```python
from build123d import *

# Parameters (mm, degrees)
BOSS_EXTRUDE1_DEPTH = 5
SKETCH2_R           = 2
CUT_EXTRUDE1_DEPTH  = 5
FILLET1_R           = 10
FILLET2_R           = 10


with BuildPart() as part:
    # Sketch1 → Boss-Extrude1 (new body)
    with BuildSketch(Plane(origin=(0, 0, 0), x_dir=(0, 0, -1), z_dir=(1, 0, 0))):
        with BuildLine():
            Line((3.89561725, -3.134352603), (36.078990527, 36.865647397))
            ThreePointArc((36.078990527, 36.865647397), (35.317725879, 43.89561725), (28.287756026, 43.134352603))
            Line((28.287756026, 43.134352603), (-3.055770002, 4.178180099))
            Line((-3.055770002, 4.178180099), (-21.704720416, -3.047928704))
            ThreePointArc((-21.704720416, -3.047928704), (-24.560430819, -9.516693509), (-18.091666014, -12.372403912))
            Line((-18.091666014, -12.372403912), (1.806527201, -4.662237604))
            Line((1.806527201, -4.662237604), (3.055770002, -4.178180099))
            Line((3.055770002, -4.178180099), (3.89561725, -3.134352603))
        make_face()
    extrude(amount=BOSS_EXTRUDE1_DEPTH)

    # Sketch2 → Cut-Extrude1 (cut)
    with BuildSketch(Plane(origin=(5, 0, 0), x_dir=(0, 0, -1), z_dir=(1, 0, 0))):
        with Locations((28.965035949, 36)):
            Circle(SKETCH2_R)
        with Locations((19.561978141, 24.313148249)):
            Circle(SKETCH2_R)
        with Locations((10.158920332, 12.626296498)):
            Circle(SKETCH2_R)
        with Locations((0.755862524, 0.939444747)):
            Circle(SKETCH2_R)
    extrude(amount=-CUT_EXTRUDE1_DEPTH, mode=Mode.SUBTRACT)

    # Fillet1
    fillet1_edges = [part.edges().sort_by_distance(p)[0] for p in [
        (2.5, 4.178180099, 3.055770002),
    ]]
    fillet(fillet1_edges, radius=FILLET1_R)

    # Fillet2
    fillet2_edges = [part.edges().sort_by_distance(p)[0] for p in [
        (2.5, -4.178180099, -3.055770002),
    ]]
    fillet(fillet2_edges, radius=FILLET2_R)


solid = part.part
```
Can you work these out from the model? Positions are in its coordinate system, mm. Coordinates: 2 decimals unless noted, no trailing zeros. Order: outer loops, then holes, each group sorted by start corner. A loop starts at its lowest first (then second) coordinate and runs counter-clockwise, first axis right, second up.
1. If we section it at A-A (y = 36): Please give me the cut outline in (x, z), then the cut area to 3 significant figures.
2. Thinking about a two-plate mould opening in Z: for faces 1 (the face through (2.54, 23.55, -21.41)), 2 (the face through (2.46, 43.83, -35.4)), 3 (the face through (2.535, 4.485, 3.234)), 4 (the face through (2.465, 17.115, -20.188)), which applies, +Z half, -Z half, draft (parallel to the pull), parting line (faces both ways), or undercut?
3. I'm going to push flat-ended pins straight in: pin 1 (3 mm diameter, centred on x = 3, z = 9, fed in from -Y); pin 2 (2 mm diameter, centred on x = 1, z = 15.5, fed in from +Y); pin 3 (1.5 mm diameter, centred on x = 4, z = 2, fed in from -Y); pin 4 (3 mm diameter, centred on y = 0.94, z = -0.76, fed in from +X). Where does each tip first touch, or does it pass through?
4. If we section it at B-B (x = 3.1): Give the number of separate pieces and of enclosed holes in the cut face, then the cut area to 3 significant figures.
5. I need wall thicknesses on line 1 (Z direction, x = 0.65, y = 11); line 2 (Z direction, x = 1.2, y = 24); line 3 (Z direction, x = 4.1, y = 42). Which ranges of each line are inside material? Lowest first, please.
Entries:
1. outline: (0, -35.38) - (5, -35.38) - (5, -30.97) - (0, -30.97) - close; (0, -26.97) - (5, -26.97) - (5, -22.55) - (0, -22.55) - close
1. area: 44.2 mm2
2. face 1: undercut
2. face 2: parting line
2. face 3: +Z half
2. face 4: -Z half
3. pin 1: stops at y = -9.43
3. pin 2: stops at y = -0.26
3. pin 3: stops at y = -6.43
3. pin 4: passes through
4. separate pieces: 1
4. enclosed holes: 4
4. area: 755 mm2
5. line 1: z = -15.27 to -11.32, -8.99 to -2.43
5. line 2: z = -25.73 to -21.54, -17.59 to -12.89
5. line 3: z = -36.77 to -27.38
